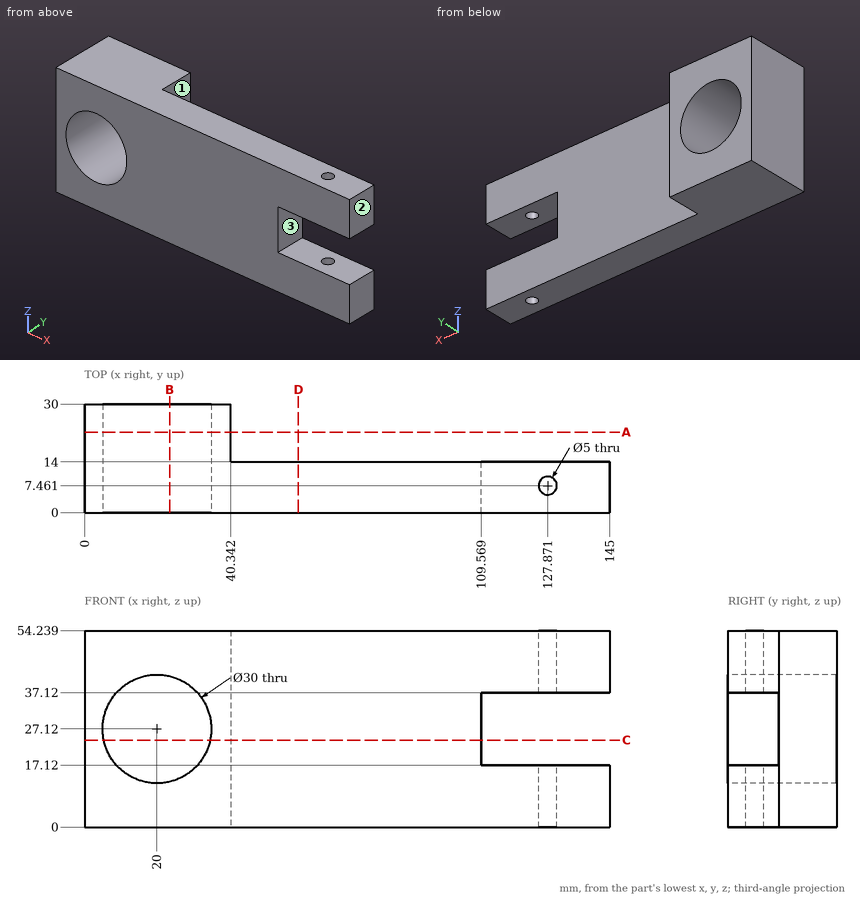
Drawing for the job (mm, zero at the part's lowest x, y, z). A direction names the side the tool comes from. Round coordinates to 2 decimals unless told otherwise and drop trailing zeros. Write each loop counter-clockwise with the first axis right and the second up, starting at its lowest first coordinate (ties: lowest second). Pieces come first, ordered by that corner, then holes. Notation, with made-up numbers: (86.25, 81) - (101.25, 81) arc R21 ccw to (101.25, 93) - close; hole circle Ø1 at (66, 52). An arc over 180 degrees is marked (long way). Use CSV: the item, a comma, the result in double quotes.
(1) Band-saw the part on C-C (z = 24). Write the cut outline in (x, y), plus the area to 3 significant figures.
Response:
outline,"(0, 0) - (5.33, 0) - (5.33, 30) - (0, 30) - close; (34.67, 0) - (109.57, 0) - (109.57, 14) - (40.34, 14) - (40.34, 30) - (34.67, 30) - close"
area,"1,300 mm²"
(2) Band-saw the part on B-B (x = 23.5). Write the cut outline in (y, z) (1 decimal).
Response:
outline,"(0, 0) - (30, 0) - (30, 12.5) - (0, 12.5) - close; (0, 41.7) - (30, 41.7) - (30, 54.2) - (0, 54.2) - close"
(3) Pin check, flat tips, straight feed: P1, Ø12, axis at x = 42.5, y = 8, coming from the -Z side; P2, Ø8, axis at x = 88.5, z = 20.5, coming from the +Y side; P3, Ø8, axis at y = 19.5, z = 18.5, coming from the +X side; P4, Ø7, axis at y = 8.5, z = 32, coming from the +X side. Stop position of each tip, or through.
Response:
P1,"z = 0"
P2,"y = 14"
P3,"x = 40.34"
P4,"x = 109.57"
(4) 3-axis set-ups, long thin cutter, end or side, ignore diameter. For the marked faces 1, 2 and 3: which of +Z, -Z, +X, -X, +Y, -Y reach the whole face in a straight line?
Response:
face 1,"+Z, -Z, +X, +Y"
face 2,"+Z, -Z, +X, +Y, -Y"
face 3,"+X, +Y, -Y"
(5) Band-saw the part on D-D (x = 59). Write the cut outline in (y, z).
Response:
outline,"(0, 0) - (14, 0) - (14, 54.24) - (0, 54.24) - close"
(6) Wall check: line 1 (X direction, y = 9.25, z = 27); line 2 (Y direction, x = 67.5, z = 21); line 3 (X direction, y = 27, z = 45). Give the ranges that are in metal, low to high.
Response:
line 1,"0 to 5, 35 to 109.57"
line 2,"0 to 14"
line 3,"0 to 40.34"
(7) Band-saw the part on A-A (y = 22.25). Write the cut outline in (x, z).
Response:
outline,"(0, 0) - (40.34, 0) - (40.34, 54.24) - (0, 54.24) - close; hole circle Ø30 at (20, 27.12)"
